from build123d import *

# Parameters (mm, degrees)
ESBO_O2_R                                    = 111.2
ESBO_O2_R_2                                  = 101.2
RESSALTO_EXTRUS_O1_DEPTH                     = 31
FURO_ROSCADO_PARA_CONDU_TE_DE_M8X1_251_REACH = 251.133
FURO_ROSCADO_PARA_CONDU_TE_DE_M8X1_251_B_R   = 4.15
FURO_ROSCADO_PARA_CONDU_TE_DE_M8X1_252_D     = 8.3
FURO_ROSCADO_PARA_CONDU_TE_DE_M8X1_252_DEPTH = 212.401
ESBO_O12_R                                   = 11.25
CORTE_EXTRUS_O1_DEPTH                        = 7.5


with BuildPart() as part:
    # Esboço2 → Ressalto-extrusão1 (new body)
    with BuildSketch(Plane.XY):
        Circle(ESBO_O2_R)
        Circle(ESBO_O2_R_2, mode=Mode.SUBTRACT)
    extrude(amount=RESSALTO_EXTRUS_O1_DEPTH)

    # Furo roscado para conduíte de M8x1.251 b (on position points) → Furo roscado para conduíte de M8x1.251 (cut, up to next)
    with BuildSketch(Plane(origin=(0, 111.2, 15.5), x_dir=(1, 0, 0), z_dir=(0, 1, 0)), mode=Mode.PRIVATE) as furo_roscado_para_condu_te_de_m8x1_251_sk1:
        Circle(FURO_ROSCADO_PARA_CONDU_TE_DE_M8X1_251_B_R)
    furo_roscado_para_condu_te_de_m8x1_251_tool1 = extrude(furo_roscado_para_condu_te_de_m8x1_251_sk1.sketch, amount=-FURO_ROSCADO_PARA_CONDU_TE_DE_M8X1_251_REACH, mode=Mode.PRIVATE) & part.part
    add(furo_roscado_para_condu_te_de_m8x1_251_tool1.solids().sort_by_distance((0, 111.2, 15.5))[0], mode=Mode.SUBTRACT)

    # Furo roscado para conduíte de M8x1.252
    with Locations(Plane(origin=(0, -111.2, 15.5), x_dir=(-1, 0, 0), z_dir=(0, -1, 0))):
        with Locations((0, 0)):
            Hole(FURO_ROSCADO_PARA_CONDU_TE_DE_M8X1_252_D / 2, depth=FURO_ROSCADO_PARA_CONDU_TE_DE_M8X1_252_DEPTH)

    # Esboço12 → Corte-extrusão1 (cut)
    with BuildSketch(Plane(origin=(111.2, 0, 0), x_dir=(0, 0, -1), z_dir=(1, 0, 0))):
        with Locations((-15.5, 0)):
            Circle(ESBO_O12_R)
    corte_extrus_o1 = extrude(amount=-CORTE_EXTRUS_O1_DEPTH, mode=Mode.SUBTRACT)

    # Espelhar1: Corte-extrusão1 across plane
    add(corte_extrus_o1.mirror(Plane(origin=(0, 0, 0), x_dir=(0, 0, 1), z_dir=(1, 0, 0))), mode=Mode.SUBTRACT)


solid = part.part
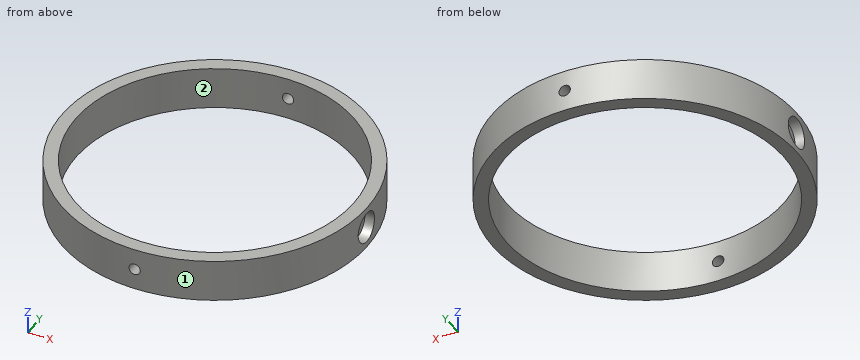
For this review, take the finished solid that the model builds, in its own axes (mm). Face numbers are marked on the shaded views. Round coordinates to 2 decimals unless told otherwise and drop trailing zeros. Loops run counter-clockwise (first coordinate to the right, second up) from the corner with the lowest first, then second, coordinate; pieces in that order, holes last. Notation, with made-up numbers: (1, 12.5) - (9, 12.5) arc R21 ccw to (9, 45.5) - close; hole circle Ø9 at (-16, 2.25). An arc over 180 degrees is marked (long way). Put each result on its own line as item: value. Start each with the question number.
1. Insertion check: P1, Ø6, axis at x = 0, z = 6, coming from the +Y side; P2, Ø10, axis at x = -78, z = 25, coming from the +Y side; P3, Ø7, axis at y = 1.5, z = 18.5, coming from the +X side; P4, Ø5, axis at x = 0, z = 15.5, coming from the -Y side. Each pin has a flat end and moves straight along its axis. Give the tip position at first contact, or say it passes through.
2. Consider section A-A on x = 0. State the section outline as (y, z) points.
3. Consider section B-B on y = -81. State the section outline as (x, z) points, plus the area to 3 significant figures.
4. Mouldability with a two-part tool opening along X and no side actions: class the marked faces 1 and 2 as +X half, -X half, draft (parallel to the pull), parting line (faces both ways), or undercut.
5. Consider section D-D on y = 0. State the section outline as (x, z) points.
6. For probe 1 along X at (y, z) = (-1, 2); probe 2 along Y at (x, z) = (75, 20); probe 3 along Y at (x, z) = (43, 12), list the stretches that pass through material, from the lowest coordinate up. Write a range as [from, to].
Result sheet:
1. P1: y = 111.2
1. P2: y = 83.88
1. P3: x = 103.7
1. P4: through
2. outline: (-111.2, 0) - (-101.2, 0) - (-101.2, 11.35) - (-111.2, 11.35) - close; (-111.2, 19.65) - (-101.2, 19.65) - (-101.2, 31) - (-111.2, 31) - close; (101.2, 0) - (111.2, 0) - (111.2, 11.35) - (101.2, 11.35) - close; (101.2, 19.65) - (111.2, 19.65) - (111.2, 31) - (101.2, 31) - close
3. outline: (-76.19, 0) - (-60.67, 0) - (-60.67, 31) - (-76.19, 31) - close; (60.67, 0) - (76.19, 0) - (76.19, 31) - (60.67, 31) - close
3. area: 962 mm^2
4. face 1: parting line
4. face 2: undercut
5. outline: (-111.2, 0) - (-101.2, 0) - (-101.2, 31) - (-111.2, 31) - (-111.2, 26.75) - (-103.7, 26.75) - (-103.7, 4.25) - (-111.2, 4.25) - close; (101.2, 0) - (111.2, 0) - (111.2, 4.25) - (103.7, 4.25) - (103.7, 26.75) - (111.2, 26.75) - (111.2, 31) - (101.2, 31) - close
6. probe 1: [-111.2, -101.2], [101.2, 111.2]
6. probe 2: [-82.1, -67.94], [67.94, 82.1]
6. probe 3: [-102.55, -91.61], [91.61, 102.55]
